from build123d import *

# Parameters (mm, degrees)
ESQUISSE1_W         = 22
ESQUISSE1_H         = 55.5
ESQUISSE1_R         = 1
ESQUISSE1_W_2       = 5
ESQUISSE1_H_2       = 5
BOSS_EXTRU_1_DEPTH  = 5
SKETCH1_W           = 22
SKETCH1_H           = 55.5
SKETCH1_W_2         = 16
SKETCH1_H_2         = 49.5
CUT_EXTRUDE1_DEPTH  = 10
SKETCH2_W           = 1
SKETCH2_H           = 5
BOSS_EXTRUDE1_DEPTH = 5
SKETCH3_R           = 1.6
CUT_EXTRUDE2_DEPTH  = 10
SKETCH4_R           = 4
SKETCH4_R_2         = 1.6
BOSS_EXTRUDE2_DEPTH = 5
SKETCH5_W           = 0.3
SKETCH5_H           = 5
CUT_EXTRUDE3_DEPTH  = 10


with BuildPart() as part:
    # Esquisse1 → Boss.-Extru.1 (new body)
    with BuildSketch(Plane.XY):
        with Locations((-6.988022113, -13.090909091)):
            Rectangle(ESQUISSE1_W, ESQUISSE1_H)
        with Locations((-6.988022113, 0.659090909)):
            Circle(ESQUISSE1_R, mode=Mode.SUBTRACT)
        with Locations((-6.988022113, -26.340909091)):
            Circle(ESQUISSE1_R, mode=Mode.SUBTRACT)
        with Locations((-12.488022113, -35.340909091)):
            Rectangle(ESQUISSE1_W_2, ESQUISSE1_H_2, mode=Mode.SUBTRACT)
        with Locations((-1.488022113, 9.159090909)):
            Rectangle(ESQUISSE1_W_2, ESQUISSE1_H_2, mode=Mode.SUBTRACT)
        with Locations((-1.488022113, -35.340909091)):
            Rectangle(ESQUISSE1_W_2, ESQUISSE1_H_2, mode=Mode.SUBTRACT)
        with Locations((-12.488022113, 9.159090909)):
            Rectangle(ESQUISSE1_W_2, ESQUISSE1_H_2, mode=Mode.SUBTRACT)
    extrude(amount=BOSS_EXTRU_1_DEPTH)

    # Sketch1 → Cut-Extrude1 (cut)
    with BuildSketch(Plane.XY.offset(5)):
        with Locations((-6.988022113, -13.090909091)):
            Rectangle(SKETCH1_W, SKETCH1_H)
        with Locations((-6.988022113, -13.090909091)):
            Rectangle(SKETCH1_W_2, SKETCH1_H_2, mode=Mode.SUBTRACT)
    extrude(amount=-CUT_EXTRUDE1_DEPTH, mode=Mode.SUBTRACT)

    # Sketch2 → Boss-Extrude1 (add)
    with BuildSketch(Plane.XY.offset(5)):
        with Locations((-3.488022113, -35.340909091)):
            Rectangle(SKETCH2_W, SKETCH2_H)
        with Locations((-10.488022113, -35.340909091)):
            Rectangle(SKETCH2_W, SKETCH2_H)
        with Locations((-3.488022113, 9.159090909)):
            Rectangle(SKETCH2_W, SKETCH2_H)
        with Locations((-10.488022113, 9.159090909)):
            Rectangle(SKETCH2_W, SKETCH2_H)
    extrude(amount=-BOSS_EXTRUDE1_DEPTH)

    # Sketch3 → Cut-Extrude2 (cut)
    with BuildSketch(Plane.XY.offset(5)):
        with Locations((-6.988022113, -35.340909091)):
            Circle(SKETCH3_R)
        with Locations((-6.988022113, 9.159090909)):
            Circle(SKETCH3_R)
    extrude(amount=-CUT_EXTRUDE2_DEPTH, mode=Mode.SUBTRACT)

    # Sketch4 → Boss-Extrude2 (add)
    with BuildSketch(Plane.XY.offset(5)):
        with Locations((-6.988022113, -35.340909091)):
            Circle(SKETCH4_R)
        with Locations((-6.988022113, -35.340909091)):
            Circle(SKETCH4_R_2, mode=Mode.SUBTRACT)
        with Locations((-6.988022113, 9.159090909)):
            Circle(SKETCH4_R)
        with Locations((-6.988022113, 9.159090909)):
            Circle(SKETCH4_R_2, mode=Mode.SUBTRACT)
    extrude(amount=-BOSS_EXTRUDE2_DEPTH)

    # Sketch5 → Cut-Extrude3 (cut)
    with BuildSketch(Plane.XY.offset(5)):
        with Locations((-3.138022113, -35.340909091)):
            Rectangle(SKETCH5_W, SKETCH5_H)
        with Locations((-10.838022113, -35.340909091)):
            Rectangle(SKETCH5_W, SKETCH5_H)
        with Locations((-3.138022113, 9.159090909)):
            Rectangle(SKETCH5_W, SKETCH5_H)
        with Locations((-10.838022113, 9.159090909)):
            Rectangle(SKETCH5_W, SKETCH5_H)
    extrude(amount=-CUT_EXTRUDE3_DEPTH, mode=Mode.SUBTRACT)


solid = part.part
For this review, take the finished solid that the model builds, in its own axes (mm). A direction names the side the tool comes from. Round coordinates to 2 decimals unless told otherwise and drop trailing zeros. Loops run counter-clockwise (first coordinate to the right, second up) from the corner with the lowest first, then second, coordinate; pieces in that order, holes last. Notation, with made-up numbers: (-31, 7.5) - (17, 7.5) arc R11 cw to (17, 13.5) - close; hole circle Ø8 at (10, 30). An arc over 180 degrees is marked (long way). Answer as CSV lines item,"result".
(1) Mouldability with a two-part tool opening along Y and no side actions: class faces 1 (the face through (-7, -13, 5)), 2 (the face through (-6.25, -36.76, 2.54)), 3 (the face through (-1, 6.659, 3)), 4 (the face through (-7.12, -25.35, 2.46)) as +Y half, -Y half, draft (parallel to the pull), parting line (faces both ways), or undercut.
Checked values:
face 1,"draft"
face 2,"undercut"
face 3,"+Y half"
face 4,"undercut"
(2) Consider section D-D on x = -9.25. Give the boundary of the cut face in (y, z).
Checked values:
outline,"(-38.64, 0) - (12.46, 0) - (12.46, 5) - (-38.64, 5) - close"
(3) Tool access review of faces 5 (the face through (-3.288, -35, 3)), 6 (the face through (-13, 6.659, 2)), 7 (the face through (-13, -32.841, 3)): name each direction out of +Z, -Z, +X, -X, +Y, -Y from which nothing blocks a thin tool from reaching the whole face with its end or side.
Checked values:
face 5,"+Z, -Z, +X, -Y"
face 6,"+Z, -Z, -X, +Y"
face 7,"+Z, -Z, -X, -Y"
(4) Insertion check: P1, Ø3, axis at x = -4, z = 1, coming from the +Y side; P2, Ø1.9, axis at x = -6.99, y = 9.16, coming from the -Z side (1 decimal); P3, Ø0.5, axis at x = -3.5, z = 3, coming from the +Y side; P4, Ø0.6, axis at x = -10.5, z = 3.5, coming from the -Y side. Each pin has a flat end and moves straight along its axis. Give the tip position at first contact, or say it passes through.
Checked values:
P1,"stops at y = 12.87"
P2,"passes through"
P3,"stops at y = 11.66"
P4,"stops at y = -37.84"
(5) Consider section C-C on x = -13. Give the boundary of the cut face in (y, z).
Checked values:
outline,"(-32.84, 0) - (6.66, 0) - (6.66, 5) - (-32.84, 5) - close"
(6) Consider section A-A on z = 0.45. Give the boundary of the cut face in (x, y), then the cut area to 3 significant figures.
Checked values:
outline,"(-14.99, -32.84) - (-10.69, -32.84) - (-10.69, -37.84) - (-10.11, -37.84) arc R4 ccw to (-3.87, -37.84) - (-3.29, -37.84) - (-3.29, -32.84) - (1.01, -32.84) - (1.01, 6.66) - (-3.29, 6.66) - (-3.29, 11.66) - (-3.87, 11.66) arc R4 ccw to (-10.11, 11.66) - (-10.69, 11.66) - (-10.69, 6.66) - (-14.99, 6.66) - close; hole circle Ø3.2 at (-6.99, -35.34); hole circle Ø3.2 at (-6.99, 9.16); hole circle Ø2 at (-6.99, -26.34); hole circle Ø2 at (-6.99, 0.66)"
area,"697 mm2"
(7) Wall thickness on line 1 (Y direction, x = -6.5, z = 1.2); line 2 (Y direction, x = -11, z = 3.95); line 3 (Y direction, x = -10.5, z = 4.4): over which ranges is each line inside the solid? List them lowest first.
Checked values:
line 1,"y = -39.31 to -36.86, -33.82 to -27.21, -25.47 to -0.21, 1.53 to 7.64, 10.68 to 13.13"
line 2,"y = -32.84 to 6.66"
line 3,"y = -37.84 to 11.66"
(8) Consider section B-B on x = -7.25. Give the boundary of the cut face in (y, z).
Checked values:
outline,"(-39.33, 0) - (-36.92, 0) - (-36.92, 5) - (-39.33, 5) - close; (-33.76, 0) - (-27.31, 0) - (-27.31, 5) - (-33.76, 5) - close; (-25.38, 0) - (-0.31, 0) - (-0.31, 5) - (-25.38, 5) - close; (1.62, 0) - (7.58, 0) - (7.58, 5) - (1.62, 5) - close; (10.74, 0) - (13.15, 0) - (13.15, 5) - (10.74, 5) - close"
